from build123d import *

# Parameters (mm, degrees)
F0_W     = 22
F0_H     = 12
F1_DEPTH = 12
F2_SIZE  = 1
F3_R     = 3.25
F3_R_2   = 1.25
F3_R_3   = 1
F4_DEPTH = 12.001
F7_R     = 2
F5_DEPTH = 4
F6_R     = 3
F8_DEPTH = 25


with BuildPart() as f1:
    # F0 (on Top) → F1 (new body)
    with BuildSketch(Plane.XY):
        Rectangle(F0_W, F0_H)
    extrude(amount=F1_DEPTH)

    # F2
    f2_edges = [f1.edges().sort_by_distance(p)[0] for p in [
        (0, -6, 12),
        (0, -6, 0),
        (0, 6, 0),
        (0, 6, 12),
    ]]
    chamfer(f2_edges, length=F2_SIZE)

    # F3 (on face) → F4 (cut, through all)
    with BuildSketch(Plane.XZ.offset(6)):
        with Locations((6.454196, 6)):
            Circle(F3_R)
        with Locations((-7.981588, 9)):
            Circle(F3_R_2)
        with Locations((-7.608019, 3)):
            Circle(F3_R_3)
    extrude(amount=-F4_DEPTH, mode=Mode.SUBTRACT)

    # F7 (on face) → F5 (cut)
    with BuildSketch(Plane.YZ.offset(11)):
        with Locations((0, 6)):
            Circle(F7_R)
    extrude(amount=-F5_DEPTH, mode=Mode.SUBTRACT)

    # F6 (on face) → F8 (cut)
    with BuildSketch(Plane.XY.offset(12)):
        with Locations((-3, 0)):
            Circle(F6_R)
    extrude(amount=-F8_DEPTH, mode=Mode.SUBTRACT)


solid = f1.part
Geometry check sheet. Reference: the model listing, model coordinates, mm. Round coordinates to 2 decimals unless told otherwise and drop trailing zeros. Order: outer loops, then holes, each group sorted by start corner. A loop starts at its lowest first (then second) coordinate and runs counter-clockwise, first axis right, second up. Notation, with made-up numbers: (46, -20.5) - (80, -20.5) arc R30 ccw to (80, 12.5) - close; hole circle Ø4 at (-22.5, 74). An arc over 180 degrees is marked (long way). One line per question, with ' | ' between items. Start each with the question number.
(1) Depth check by flat-ended pin: pin 1 Ø2.5 at (x, z) = (-7.61, 3) entering from +Y. Enter the tip coordinate at first touch or a pass-through.
(2) Sectioned sample at D-D on z = 3. Record the cut outline in (x, y).
(3) Sectioned sample at A-A on y = 0. Record the cut outline in (x, z).
(4) Thickness scan on L1, parallel to Z at x = 10.35, y = 0; L2, parallel to X at y = 2, z = 8.75; L3, parallel to X at y = -3.5, z = 8. Record the ranges inside material, lowest first. Write a range as [from, to].
(5) Sectioned sample at B-B on z = 10. Record the cut outline in (x, y).
(6) Sectioned sample at C-C on x = -3. Record the cut outline in (y, z).
(7) Release check for a two-part mould opening along Y. For faces 1 (the flat face through (-0.2, -5.5, 0.5)), 2 (the flat face through (-0.2, 5.5, 11.5)), 3 (the cylindrical face through (10, -2, 6)) record: released by +Y, released by -Y, zero draft, split by the parting line, or undercut.
Conclusion:
1) pin 1: stops at y = 6
2) outline: (-11, -6) - (-8.61, -6) - (-8.61, 6) - (-11, 6) - close; (-6.61, -6) - (5.2, -6) - (5.2, 6) - (-6.61, 6) - close; (7.7, -6) - (11, -6) - (11, 6) - (7.7, 6) - close; hole circle Ø6 at (-3, 0)
3) outline: (-11, 0) - (-6, 0) - (-6, 12) - (-11, 12) - close; (0, 0) - (11, 0) - (11, 4) - (9.02, 4) arc R3.25 cw (long way) to (9.02, 8) - (11, 8) - (11, 12) - (0, 12) - close; hole circle Ø2.5 at (-7.98, 9); hole circle Ø2 at (-7.61, 3)
4) L1: z = [0, 4], [8, 12] | L2: x = [-11, -9.21], [-6.76, -5.24], [-0.76, 4.72], [8.19, 11] | L3: x = [-11, -8.73], [-7.23, 3.89], [9.02, 11]
5) outline: (-11, -6) - (-8.73, -6) - (-8.73, 6) - (-11, 6) - close; (-7.23, -6) - (11, -6) - (11, 6) - (-7.23, 6) - close; hole circle Ø6 at (-3, 0)
6) outline: (-6, 1) - (-5, 0) - (-3, 0) - (-3, 12) - (-5, 12) - (-6, 11) - close; (3, 0) - (5, 0) - (6, 1) - (6, 11) - (5, 12) - (3, 12) - close
7) face 1: released by -Y | face 2: released by +Y | face 3: undercut
